```python
from build123d import *

# Parameters (mm, degrees)
SKETCH_1_W          = 15
SKETCH_1_H          = 15
EXTRUDE_1_DEPTH     = 3
FILLET_1_R          = 1
SKETCH_2_R          = 0.75
CUT_EXTRUDE_1_DEPTH = 4
SKETCH_3_R          = 6.839868167
CUT_EXTRUDE_2_DEPTH = 1


with BuildPart() as part:
    # 草图1 → 凸台-拉伸1 (new body)
    with BuildSketch(Plane(origin=(0, 0, 0), x_dir=(1, 0, 0), z_dir=(0, 1, 0))):
        Rectangle(SKETCH_1_W, SKETCH_1_H)
    extrude(amount=EXTRUDE_1_DEPTH)

    # 圆角1
    fillet_1_edges = [part.edges().sort_by_distance(p)[0] for p in [
        (-7.5, 1.5, -7.5),
        (7.5, 1.5, -7.5),
        (7.5, 1.5, 7.5),
        (-7.5, 1.5, 7.5),
    ]]
    fillet(fillet_1_edges, radius=FILLET_1_R)

    # 草图2 → 切除-拉伸1 (cut, through all)
    with BuildSketch(Plane(origin=(0, 3, 0), x_dir=(1, 0, 0), z_dir=(0, 1, 0))):
        with Locations((-6.25, -6.25)):
            Circle(SKETCH_2_R)
        with Locations((6.25, 6.25)):
            Circle(SKETCH_2_R)
    extrude(amount=-CUT_EXTRUDE_1_DEPTH, mode=Mode.SUBTRACT)

    # 草图3 → 切除-拉伸2 (cut)
    with BuildSketch(Plane(origin=(0, 3, 0), x_dir=(1, 0, 0), z_dir=(0, 1, 0))):
        Circle(SKETCH_3_R)
    extrude(amount=-CUT_EXTRUDE_2_DEPTH, mode=Mode.SUBTRACT)


solid = part.part
```
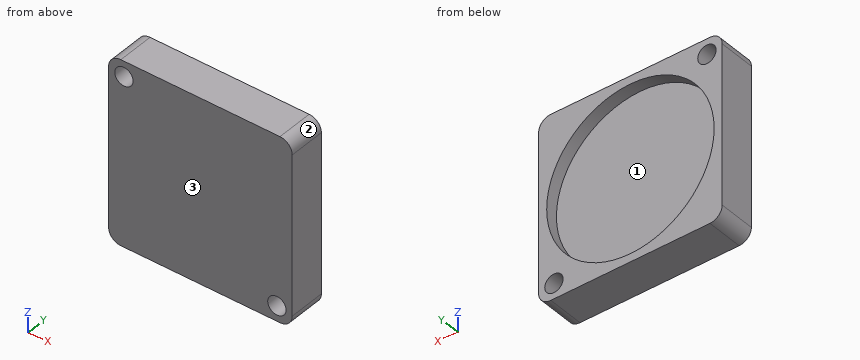
For this review, take the finished solid that the model builds, in its own axes (mm). Face numbers are marked on the shaded views. Round coordinates to 2 decimals unless told otherwise and drop trailing zeros. Write each loop counter-clockwise with the first axis right and the second up, starting at its lowest first coordinate (ties: lowest second). Pieces come first, ordered by that corner, then holes. Notation, with made-up numbers: (49.5, -17) - (105.5, -17) arc R30 cw to (105.5, 15) - close; hole circle Ø11 at (20.5, 11). An arc over 180 degrees is marked (long way). Use CSV: the item, a comma, the result in double quotes.
1) Add section D-D on x = -5.75. Write out the cut boundary in (y, z).
Conclusion:
outline,"(0, -7.5) - (3, -7.5) - (3, -3.7) - (2, -3.7) - (2, 3.7) - (3, 3.7) - (3, 5.69) - (0, 5.69) - close; (0, 6.81) - (3, 6.81) - (3, 7.5) - (0, 7.5) - close"
2) Add section A-A on x = 0. Write out the cut boundary in (y, z), and give its area (3 significant figures).
Conclusion:
outline,"(0, -7.5) - (3, -7.5) - (3, -6.84) - (2, -6.84) - (2, 6.84) - (3, 6.84) - (3, 7.5) - (0, 7.5) - close"
area,"31.3 mm^2"
3) Clearance check with a flat-ended pin moving along its axis: pin 1 Ø2 at (x, z) = (2, -2) entering from +Y. State where the tip first meets the part, or that it passes through.
Conclusion:
pin 1,"stops at y = 2"
4) Add section B-B on z = 6.25. Write out the cut boundary in (x, y).
Conclusion:
outline,"(-7.5, 0) - (-7, 0) - (-7, 3) - (-7.5, 3) - close; (-5.5, 0) - (7.5, 0) - (7.5, 3) - (2.78, 3) - (2.78, 2) - (-2.78, 2) - (-2.78, 3) - (-5.5, 3) - close"
5) Wall thickness on line 1 along Z through (x, y) = (6.25, 1.45); line 2 along Z through (x, y) = (-6.25, 0.9); line 3 along X through (y, z) = (2.1, 6.25): over which ranges is each line inside the solid? List them lowest first. Write a range as from..to.
Conclusion:
line 1,"z = -7.5..-7, -5.5..7.5"
line 2,"z = -7.5..5.5, 7..7.5"
line 3,"x = -7.5..-7, -5.5..-2.78, 2.78..7.5"
6) The part is to be moulded in two halves that separate along Y. For the marked faces 1, 2 and 3, say which applies: pulls with the +Y half, pulls with the -Y half, needs draft (parallel to the pull), parting line crosses it, or undercut.
Conclusion:
face 1,"pulls with the +Y half"
face 2,"needs draft"
face 3,"pulls with the -Y half"
7) Add section C-C on y = 1.2. Write out the cut boundary in (x, z), and give its area (3 significant figures).
Conclusion:
outline,"(-7.5, -6.5) arc R1 ccw to (-6.5, -7.5) - (6.5, -7.5) arc R1 ccw to (7.5, -6.5) - (7.5, 6.5) arc R1 ccw to (6.5, 7.5) - (-6.5, 7.5) arc R1 ccw to (-7.5, 6.5) - close; hole circle Ø1.5 at (-6.25, 6.25); hole circle Ø1.5 at (6.25, -6.25)"
area,"221 mm^2"
